Work out the finished part from the listing and answer in its coordinate system (mm). Coordinates: 2 decimals unless noted, no trailing zeros. Write each loop counter-clockwise with the first axis right and the second up, starting at its lowest first coordinate (ties: lowest second). Pieces come first, ordered by that corner, then holes. Notation, with made-up numbers: (79.25, 63) - (138.25, 63) arc R29 ccw to (138.25, 99) - close; hole circle Ø1 at (-25.75, 9.5). An arc over 180 degrees is marked (long way). One line per item, written item: value.
```python
from build123d import *

# Parameters (mm, degrees)
SKETCH_1_W          = 30
SKETCH_1_H          = 10
SKETCH_1_R          = 1.5
EXTRUDE_1_DEPTH     = 2
SKETCH_4_R          = 1.5
EXTRUDE_3_DEPTH     = 2
SKETCH_5_R          = 1.5
CUT_EXTRUDE_2_DEPTH = 42.397139466


with BuildPart() as part:
    # 草图1 → 凸台-拉伸1 (new body)
    with BuildSketch(Plane.XY):
        with Locations((10, 0)):
            Rectangle(SKETCH_1_W, SKETCH_1_H)
        Circle(SKETCH_1_R, mode=Mode.SUBTRACT)
        with Locations((20, 0)):
            Circle(SKETCH_1_R, mode=Mode.SUBTRACT)
    extrude(amount=EXTRUDE_1_DEPTH)

    # 草图4 → 凸台-拉伸3 (add)
    # profile 1 of 3: a face of its own
    with BuildSketch(Plane(origin=(0, 0, 0), x_dir=(-1, 0, 0), z_dir=(0, 0, -1))):
        with BuildLine():
            Line((-30.725715478, -22.717516962), (-20.496502291, -5))
            Line((-20.496502291, -5), (-13.568299061, -5))
            Line((-13.568299061, -5), (-25.529563056, -25.717516962))
            ThreePointArc((-25.529563056, -25.717516962), (-29.627639267, -26.815593174), (-30.725715478, -22.717516962))
        make_face()
        with Locations((-28.127639267, -24.217516962)):
            Circle(SKETCH_4_R, mode=Mode.SUBTRACT)
    # profile 2 of 3: a face of its own
    with BuildSketch(Plane(origin=(0, 0, 0), x_dir=(-1, 0, 0), z_dir=(0, 0, -1))):
        with BuildLine():
            Line((-14.674826287, 5), (-12.937385919, 5))
            ThreePointArc((-12.937385919, 5), (-11.863593392, 5.452636831), (-10.789800864, 5))
            Line((-10.789800864, 5), (-9.052360496, 5))
            ThreePointArc((-9.052360496, 5), (-11.863593392, 6.952636831), (-14.674826287, 5))
        make_face()
    # profile 3 of 3: a face of its own
    with BuildSketch(Plane(origin=(0, 0, 0), x_dir=(-1, 0, 0), z_dir=(0, 0, -1))):
        with BuildLine():
            Line((5, 5), (9.052360496, 5))
            ThreePointArc((9.052360496, 5), (11.613435505, 6.942188809), (14.461669603, 5.452636831))
            Line((14.461669603, 5.452636831), (30.725715478, -22.717516962))
            ThreePointArc((30.725715478, -22.717516962), (29.627639267, -26.815593174), (25.529563056, -25.717516962))
            Line((25.529563056, -25.717516962), (13.568299061, -5))
            Line((13.568299061, -5), (5, -5))
            Line((5, -5), (5, 5))
        make_face()
        with Locations((11.863593392, 3.952636831)):
            Circle(SKETCH_4_R, mode=Mode.SUBTRACT)
        with Locations((28.127639267, -24.217516962)):
            Circle(SKETCH_4_R, mode=Mode.SUBTRACT)
    extrude(amount=-EXTRUDE_3_DEPTH)

    # 草图5 → 切除-拉伸2 (cut, through all)
    with BuildSketch(Plane(origin=(0, 0, 0), x_dir=(-1, 0, 0), z_dir=(0, 0, -1))):
        with Locations((-11.863593392, 3.952636831)):
            Circle(SKETCH_5_R)
    extrude(amount=-CUT_EXTRUDE_2_DEPTH, mode=Mode.SUBTRACT)


solid = part.part
```
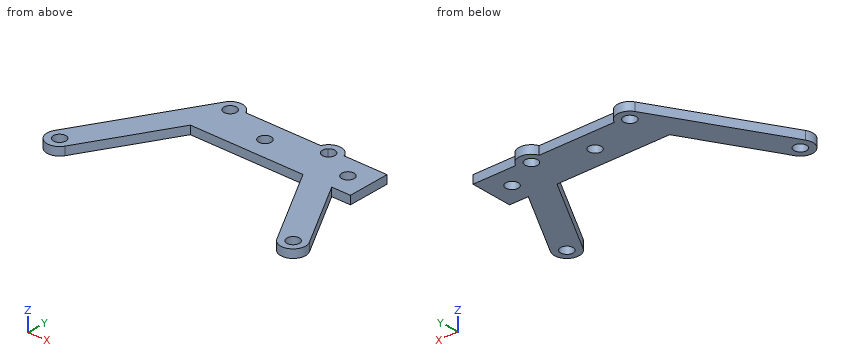
Item 1: Section B-B, the plane y = -16 is taken. Determine the outline of the cut face in (x, z).
Evaluation:
outline: (-26.85, 0) - (-19.92, 0) - (-19.92, 2) - (-26.85, 2) - close; (19.92, 0) - (26.85, 0) - (26.85, 2) - (19.92, 2) - close
Item 2: Given pin 1 (0.6 mm diameter, centred on x = -2, z = 0.5, fed in from -Y); pin 2 (1 mm diameter, centred on y = -9, z = 1, fed in from +X), each flat-ended and moving along its own axis, determine where each tip first touches the part or whether it passes through.
Evaluation:
pin 1: stops at y = -5
pin 2: stops at x = 23.09
Item 3: Section D-D, the plane y = 0 is taken. Determine the outline of the cut face in (x, z), then the cut area to 3 significant figures.
Evaluation:
outline: (-17.61, 0) - (-1.5, 0) - (-1.5, 2) - (-17.61, 2) - close; (1.5, 0) - (18.5, 0) - (18.5, 2) - (1.5, 2) - close; (21.5, 0) - (25, 0) - (25, 2) - (21.5, 2) - close
area: 73.2 mm2
Item 4: Section A-A, the plane x = 0 is taken. Determine the outline of the cut face in (y, z).
Evaluation:
outline: (-5, 0) - (-1.5, 0) - (-1.5, 2) - (-5, 2) - close; (1.5, 0) - (5, 0) - (5, 2) - (1.5, 2) - close
Item 5: Consider probe 1 along X at (y, z) = (-23, 0.1); probe 2 along Y at (x, z) = (0, 0.55); probe 3 along Y at (x, z) = (-2, 1.7). Determine where each line is inside the solid, lowest interval first.
Evaluation:
probe 1: x = -30.87 to -29, -27.25 to -23.96, 23.96 to 27.25, 29 to 30.87
probe 2: y = -5 to -1.5, 1.5 to 5
probe 3: y = -5 to 5
Item 6: Section C-C, the plane z = 0.5 is taken. Determine the outline of the cut face in (x, y), then the cut area to 3 significant figures.
Evaluation:
outline: (-30.73, -22.72) arc R3 ccw to (-25.53, -25.72) - (-13.57, -5) - (13.57, -5) - (25.53, -25.72) arc R3 ccw to (30.73, -22.72) - (20.5, -5) - (25, -5) - (25, 5) - (14.67, 5) arc R3 ccw to (9.05, 5) - (-9.05, 5) arc R3 ccw to (-14.46, 5.45) - close; hole circle Ø3 at (-28.13, -24.22); hole circle Ø3 at (-11.86, 3.95); hole circle Ø3 at (0, 0); hole circle Ø3 at (11.86, 3.95); hole circle Ø3 at (20, 0); hole circle Ø3 at (28.13, -24.22)
area: 694 mm2
